from build123d import *

# Parameters (mm, degrees)
SKETCH1_W           = 57.15
SKETCH1_H           = 57.15
SKETCH1_R           = 3.175
SKETCH1_R_2         = 11.3
BOSS_EXTRUDE1_DEPTH = 2.032
BOSS_EXTRUDE2_START = 2.032
SKETCH1_2_W         = 57.15
SKETCH1_2_H         = 57.15
SKETCH1_2_R         = 11.3
SKETCH1_2_R_2       = 3.175
BOSS_EXTRUDE2_DEPTH = 2.54


with BuildPart() as part:
    # Sketch1 → Boss-Extrude1 (new body)
    with BuildSketch(Plane.XY):
        Rectangle(SKETCH1_W, SKETCH1_H)
        with Locations((-16.522101848, 16.522101848)):
            Circle(SKETCH1_R, mode=Mode.SUBTRACT)
        with Locations((16.522101848, 16.522101848)):
            Circle(SKETCH1_R, mode=Mode.SUBTRACT)
        with Locations((16.522101848, -16.522101848)):
            Circle(SKETCH1_R, mode=Mode.SUBTRACT)
        with Locations((-16.522101848, -16.522101848)):
            Circle(SKETCH1_R, mode=Mode.SUBTRACT)
        Circle(SKETCH1_R_2, mode=Mode.SUBTRACT)
    extrude(amount=BOSS_EXTRUDE1_DEPTH)

    # Sketch1<2> → Boss-Extrude2 (add)
    # profile 1 of 2: a face of its own
    with BuildSketch(Plane.XY.offset(BOSS_EXTRUDE2_START)):
        Rectangle(SKETCH1_2_W, SKETCH1_2_H)
        Circle(SKETCH1_2_R, mode=Mode.SUBTRACT)
        with Locations(Location((-16.522101848, -16.522101848, 0), (0, 0, 180))):
            Circle(SKETCH1_2_R_2, mode=Mode.SUBTRACT)
        with Locations(Location((16.522101848, -16.522101848, 0), (0, 0, 180))):
            Circle(SKETCH1_2_R_2, mode=Mode.SUBTRACT)
        with Locations(Location((16.522101848, 16.522101848, 0), (0, 0, 180))):
            Circle(SKETCH1_2_R_2, mode=Mode.SUBTRACT)
        with Locations(Location((-16.522101848, 16.522101848, 0), (0, 0, 180))):
            Circle(SKETCH1_2_R_2, mode=Mode.SUBTRACT)
    # profile 2 of 2: a face of its own
    with BuildSketch(Plane.XY.offset(BOSS_EXTRUDE2_START)):
        Circle(SKETCH1_2_R)
    extrude(amount=BOSS_EXTRUDE2_DEPTH)


solid = part.part
Read the model definition and answer for the solid it produces. Units are mm, in the model's axes. A direction names the side the tool comes from. Round coordinates to 2 decimals unless told otherwise and drop trailing zeros. Order: outer loops, then holes, each group sorted by start corner. A loop starts at its lowest first (then second) coordinate and runs counter-clockwise, first axis right, second up.
1) The part is cut by section A-A on y = 0. Write down the section's boundary in (x, z) (3 decimals), plus the area to 3 significant figures.
2) The mould has two halves that part along Y. Classify faces 3 (the face through (16.731, -13.354, 1.746)), 4 (the face through (-28.575, 0, 2)), 5 (the face through (-16.31, 19.69, 1.75)), 6 (the face through (0, 28.575, 2)): released by +Y, released by -Y, zero draft, split by the parting line, or undercut.
3) Straight lines are drawn through the part: L1, parallel to X at y = -19, z = 3.4 (3 decimals); L2, parallel to Y at x = 0, z = 1.35 (3 decimals); L3, parallel to X at y = -14, z = 2.7 (3 decimals). For each, find the intervals that lie inside material, in ascending order.
4) For faces 1 (the face through (10.78, 3.39, 1)), 2 (the face through (0, -28.575, 2)), determine the directions among +Z, -Z, +X, -X, +Y, -Y from which every point of the face is accessible in a straight line to the end or side of a thin tool.
5) The part is cut by section C-C on y = 14. Write down the section's boundary in (x, z) (3 decimals).
Resolved:
1. outline: (-28.575, 0) - (-11.3, 0) - (-11.3, 2.032) - (11.3, 2.032) - (11.3, 0) - (28.575, 0) - (28.575, 4.572) - (-28.575, 4.572) - close
1. area: 215 mm2
2. face 3: undercut
2. face 4: zero draft
2. face 5: undercut
2. face 6: released by +Y
3. L1: x = -28.575 to -18.507, -14.537 to 14.537, 18.507 to 28.575
3. L2: y = -28.575 to -11.3, 11.3 to 28.575
3. L3: x = -28.575 to -18.451, -14.593 to 14.593, 18.451 to 28.575
4. face 1: -Z
4. face 2: +Z, -Z, +X, -X, -Y
5. outline: (-28.575, 0) - (-18.451, 0) - (-18.451, 4.572) - (-28.575, 4.572) - close; (-14.593, 0) - (14.593, 0) - (14.593, 4.572) - (-14.593, 4.572) - close; (18.451, 0) - (28.575, 0) - (28.575, 4.572) - (18.451, 4.572) - close
